The model under review builds one solid part; all positions refer to its coordinate system, in mm. A direction names the side the tool comes from. Coordinates: 2 decimals unless noted, no trailing zeros. Write each loop counter-clockwise with the first axis right and the second up, starting at its lowest first coordinate (ties: lowest second). Pieces come first, ordered by that corner, then holes.
1) Mouldability with a two-part tool opening along Z and no side actions: class faces 4 (the cylindrical face through (-2475.174, -604.285, 890.549)), 5 (the flat face through (-2493, -1219.2, 910)) as released by +Z, released by -Z, zero draft, split by the parting line, or undercut.
2) Add section B-B, the plane z = 859. State the section outline as (x, y) points, then the cut area to 3 significant figures.
3) Add section C-C, the plane y = -517.5. State the section outline as (x, z) points (3 decimals).
4) Machinability: for faces 1 (the cylindrical face through (-2492.73, -603, 883.61)), 2 (the flat face through (-2493.4, -1219.2, 827.1)), 3 (the flat face through (-2491, -3.81, 856)), which of the approach directions +Z, -Z, +X, -X, +Y, -Y give a long, thin tool a straight path to every point of the face, cutting with its end or side? Answer none if there is none.
5) For P1, Ø10, axis at x = -2511.5, z = 806, coming from the -Y side; P2, Ø2, axis at y = -440.5, z = 813.5, coming from the -X side; P3, Ø4, axis at y = -224, z = 896, coming from the +X side; P4, Ø10, axis at x = -2451.64, z = 793.44, coming from the +Y side, all flat-tipped, find the tip position at first contact; note any pin that passes through.
6) For line 1 (Y direction, x = -2497.5, z = 885.5); line 2 (Y direction, x = -2460, z = 786); line 3 (X direction, y = -1034, z = 896), list the stretches that pass through material, from the lowest coordinate up.
7) Add section A-A, the plane x = -2489.5. State the section outline as (y, z) points.
from build123d import *

# Parameters (mm, degrees)
F0_W     = 101.6
F0_H     = 152.4
F0_R     = 15.875
F0_R_2   = 6.35
F1_DEPTH = 6.35
F2_DEPTH = 1219.2
F3_T     = -2.54


with BuildPart() as f1:
    # F0 (on Front) → F1 (new body)
    with BuildSketch(Plane.XZ):
        with Locations((-2489.8389577866, 855.3545203808)):
            Rectangle(F0_W, F0_H)
        with Locations((-2489.8389577866, 814.0795203808)):
            Circle(F0_R, mode=Mode.SUBTRACT)
        with Locations((-2451.6389285668, 793.4423906328)):
            Circle(F0_R_2, mode=Mode.SUBTRACT)
        with Locations((-2527.7759553845, 917.5029841941)):
            Circle(F0_R_2, mode=Mode.SUBTRACT)
        with Locations((-2489.8389577866, 896.6295203808)):
            Circle(F0_R, mode=Mode.SUBTRACT)
    extrude(amount=F1_DEPTH)

    # F0 (on Front) → F2 (join)
    with BuildSketch(Plane.XZ):
        with Locations((-2489.8389577866, 896.6295203808)):
            Circle(F0_R)
        with Locations((-2489.8389577866, 814.0795203808)):
            Circle(F0_R)
    extrude(amount=F2_DEPTH)

    # F3
    f3_openings = [f1.faces().sort_by_distance(p)[0] for p in [
        (-2489.838958, -1219.2, 896.62952),
        (-2489.838958, -1219.2, 814.07952),
    ]]
    offset(amount=F3_T, openings=f3_openings, kind=Kind.INTERSECTION)


solid = f1.part
Geometry results:
1. face 4: undercut
1. face 5: zero draft
2. outline: (-2540.64, -6.35) - (-2439.04, -6.35) - (-2439.04, 0) - (-2540.64, 0) - close; hole (-2538.1, -3.81) - (-2441.58, -3.81) - (-2441.58, -2.54) - (-2538.1, -2.54) - close
2. area: 523 mm2
3. outline: circle Ø31.75 at (-2489.839, 814.08); circle Ø31.75 at (-2489.839, 896.63); hole circle Ø26.67 at (-2489.839, 814.08); hole circle Ø26.67 at (-2489.839, 896.63)
4. face 1: -Y
4. face 2: +Z, -Z, +X, -X, -Y
4. face 3: none
5. P1: stops at y = -6.35
5. P2: stops at x = -2505.71
5. P3: stops at x = -2473.96
5. P4: passes through
6. line 1: y = -1219.2 to -3.81, -2.54 to 0
6. line 2: y = -6.35 to -3.81, -2.54 to 0
6. line 3: x = -2505.7 to -2503.16, -2476.52 to -2473.98
7. outline: (-1219.2, 798.21) - (-6.35, 798.21) - (-6.35, 779.15) - (0, 779.15) - (0, 931.55) - (-6.35, 931.55) - (-6.35, 912.5) - (-1219.2, 912.5) - (-1219.2, 909.96) - (-3.81, 909.96) - (-3.81, 929.01) - (-2.54, 929.01) - (-2.54, 781.69) - (-3.81, 781.69) - (-3.81, 800.75) - (-1219.2, 800.75) - close; (-1219.2, 827.41) - (-3.81, 827.41) - (-3.81, 883.3) - (-1219.2, 883.3) - (-1219.2, 880.76) - (-6.35, 880.76) - (-6.35, 829.95) - (-1219.2, 829.95) - close
